For this review, take the finished solid that the model builds, in its own axes (mm). Face numbers are marked on the shaded views. A direction names the side the tool comes from. Coordinates: 2 decimals unless noted, no trailing zeros. Write each loop counter-clockwise with the first axis right and the second up, starting at its lowest first coordinate (ties: lowest second). Pieces come first, ordered by that corner, then holes.
```python
from build123d import *

# Parameters (mm, degrees)
SKETCH1_W                       = 30
SKETCH1_H                       = 18
BOSS_EXTRUDE1_DEPTH             = 1.5
BOSS_EXTRUDE2_DEPTH             = 3.5
SKETCH3_W                       = 3
SKETCH3_H                       = 5
BOSS_EXTRUDE3_DEPTH             = 0.35
SKETCH4_R                       = 0.875
BOSS_EXTRUDE4_DEPTH             = 7.5
BOSS_EXTRUDE4_DIRECTION_2_REACH = 33.718


with BuildPart() as part:
    # Sketch1 → Boss-Extrude1 (new body)
    with BuildSketch(Plane.XY):
        Rectangle(SKETCH1_W, SKETCH1_H)
    extrude(amount=BOSS_EXTRUDE1_DEPTH)

    # Sketch2 → Boss-Extrude2 (add)
    with BuildSketch(Plane.XY.offset(1.5)):
        with BuildLine():
            Line((-4, -1.1), (4, -1.1))
            ThreePointArc((4, -1.1), (4.707106781, -0.807106781), (5, -0.1))
            Line((5, -0.1), (5, 7.9))
            ThreePointArc((5, 7.9), (4.707106781, 8.607106781), (4, 8.9))
            Line((4, 8.9), (-4, 8.9))
            ThreePointArc((-4, 8.9), (-4.707106781, 8.607106781), (-5, 7.9))
            Line((-5, 7.9), (-5, -0.1))
            ThreePointArc((-5, -0.1), (-4.707106781, -0.807106781), (-4, -1.1))
        make_face()
    extrude(amount=BOSS_EXTRUDE2_DEPTH)

    # Sketch3 → Boss-Extrude3 (add)
    with BuildSketch(Plane.XY.offset(1.5)):
        with Locations((-13.4, 6.4)):
            Rectangle(SKETCH3_W, SKETCH3_H)
        with Locations((-13.4, -6.4)):
            Rectangle(SKETCH3_W, SKETCH3_H)
    boss_extrude3 = extrude(amount=BOSS_EXTRUDE3_DEPTH)

    # Sketch4 → Boss-Extrude4 (add)
    with BuildSketch(Plane.ZY.offset(15)):
        with Locations((0.975, 6.4)):
            Circle(SKETCH4_R)
        with Locations((0.975, -6.4)):
            Circle(SKETCH4_R)
    boss_extrude4 = extrude(amount=BOSS_EXTRUDE4_DEPTH)

    # Boss-Extrude4 direction 2: up to this face of the body (flat: up to its plane)
    boss_extrude4_direction_2_end = Plane(part.part.faces().sort_by_distance((-14.9, -6.4, 1.675))[0])
    # Sketch4 → Boss-Extrude4 direction 2 (add, up to the picked face)
    with BuildSketch(Plane.ZY.offset(15), mode=Mode.PRIVATE) as boss_extrude4_direction_2_sk1:
        with Locations((0.975, 6.4)):
            Circle(SKETCH4_R)
    boss_extrude4_direction_2_tool1 = split(extrude(boss_extrude4_direction_2_sk1.sketch, amount=-BOSS_EXTRUDE4_DIRECTION_2_REACH, mode=Mode.PRIVATE), bisect_by=boss_extrude4_direction_2_end, keep=Keep.BOTH, mode=Mode.PRIVATE)
    # Sketch4 → Boss-Extrude4 direction 2 (add, up to the picked face)
    with BuildSketch(Plane.ZY.offset(15), mode=Mode.PRIVATE) as boss_extrude4_direction_2_sk2:
        with Locations((0.975, -6.4)):
            Circle(SKETCH4_R)
    boss_extrude4_direction_2_tool2 = split(extrude(boss_extrude4_direction_2_sk2.sketch, amount=-BOSS_EXTRUDE4_DIRECTION_2_REACH, mode=Mode.PRIVATE), bisect_by=boss_extrude4_direction_2_end, keep=Keep.BOTH, mode=Mode.PRIVATE)
    boss_extrude4_direction_2_1 = boss_extrude4_direction_2_tool1.solids().sort_by(Axis((-15, 6.4, 0.975), (1, 0, 0)))[0]
    add(boss_extrude4_direction_2_1)
    boss_extrude4_direction_2_2 = boss_extrude4_direction_2_tool2.solids().sort_by(Axis((-15, -6.4, 0.975), (1, 0, 0)))[0]
    add(boss_extrude4_direction_2_2)
    boss_extrude4_direction_2 = boss_extrude4_direction_2_1 + boss_extrude4_direction_2_2  # Boss-Extrude4 direction 2 as one shape, for the pattern or mirror that repeats it

    # Mirror2: Boss-Extrude3, Boss-Extrude4, Boss-Extrude4 direction 2 across plane
    add(boss_extrude3.mirror(Plane(origin=(0, 0, 0), x_dir=(0, 0, 1), z_dir=(1, 0, 0))))
    add(boss_extrude4.mirror(Plane(origin=(0, 0, 0), x_dir=(0, 0, 1), z_dir=(1, 0, 0))))
    add(boss_extrude4_direction_2.mirror(Plane(origin=(0, 0, 0), x_dir=(0, 0, 1), z_dir=(1, 0, 0))))


solid = part.part
```
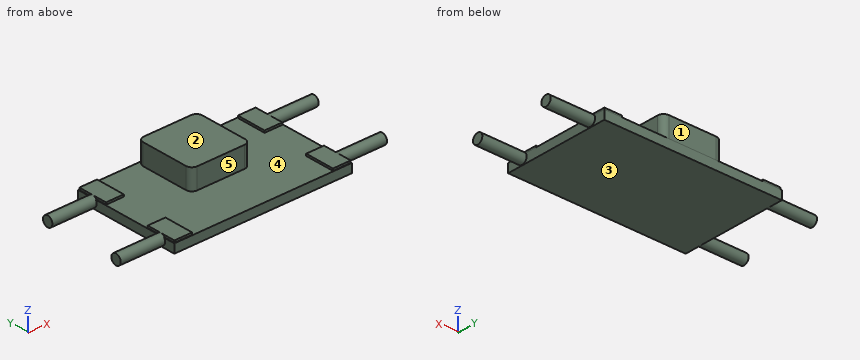
1) Tool access review of the marked faces 1 and 2: name each direction out of +Z, -Z, +X, -X, +Y, -Y from which nothing blocks a thin tool from reaching the whole face with its end or side.
2) Consider section D-D (y = -3.5). Give the boundary of the cut face in (x, z).
3) Consider section C-C (y = 1). Give the boundary of the cut face in (x, z).
4) Clearance check with flat-ended pins moving along their axes: P1, Ø3.5, axis at x = 13.5, y = 6, coming from the +Z side; P2, Ø1.5, axis at x = -0.5, z = 2.5, coming from the -Y side; P3, Ø1, axis at x = 1, z = 3.5, coming from the +Y side. State where each tip first meets the part, or that it passes through.
5) Consider section B-B (x = 19). Give the boundary of the cut face in (y, z) (3 decimals), then the cut area to 3 significant figures.
6) Consider section A-A (x = 1). Give the boundary of the cut face in (y, z), then the cut area to 3 significant figures.
7) The part is to be moulded in two halves that separate along Y. For the marked faces 3, 4 and 5, say which applies: pulls with the +Y half, pulls with the -Y half, needs draft (parallel to the pull), parting line crosses it, or undercut.
8) For L1, parallel to X at y = 6.5, z = 1.7; L2, parallel to X at y = 2.75, z = 2.2; L3, parallel to Z at x = 14, y = -7.5, list the stretches that pass through material, from the lowest coordinate up.
Results:
1. face 1: +Z, +X, -X, +Y
1. face 2: +Z, +X, -X, +Y, -Y
2. outline: (-15, 0) - (15, 0) - (15, 1.5) - (-15, 1.5) - close
3. outline: (-15, 0) - (15, 0) - (15, 1.5) - (5, 1.5) - (5, 5) - (-5, 5) - (-5, 1.5) - (-15, 1.5) - close
4. P1: stops at z = 1.85
4. P2: stops at y = -1.1
4. P3: stops at y = 8.9
5. outline: circle Ø1.75 at (-6.4, 0.975); circle Ø1.75 at (6.4, 0.975)
5. area: 4.81 mm2
6. outline: (-9, 0) - (9, 0) - (9, 1.5) - (8.9, 1.5) - (8.9, 5) - (-1.1, 5) - (-1.1, 1.5) - (-9, 1.5) - close
6. area: 62.0 mm2
7. face 3: needs draft
7. face 4: undercut
7. face 5: pulls with the -Y half
8. L1: x = -22.5 to -11.9, -5 to 5, 11.9 to 22.5
8. L2: x = -5 to 5
8. L3: z = 0 to 1.85
